```python
from build123d import *

# Parameters (mm, degrees)
F1_DEPTH = 19.05
F2_W     = 6.35
F2_H     = 4.7625
F2_W_2   = 50.8
F3_DEPTH = 63.5
F5_DEPTH = 10.16


with BuildPart() as f1:
    # F0 (on Front) → F1 (new body)
    with BuildSketch(Plane.XZ):
        Polygon((0, -38.1), (0, 0), (0, 38.1), (-38.1, 38.1), (-38.1, 0), (-38.1, -38.1), align=None)
        Polygon((0, 38.1), (0, 0), (0, -38.1), (38.1, -38.1), (38.1, 0), (38.1, 38.1), align=None)
    extrude(amount=F1_DEPTH)

    # F2 (on face) → F3 (cut)
    with BuildSketch(Plane.XY.offset(38.1)):
        Polygon((-25.4, -14.2875), (25.4, -14.2875), (25.4, -9.525), (25.4, -4.7625), (-25.4, -4.7625), (-25.4, -9.525), align=None)
        with Locations((28.575, -11.90625)):
            Rectangle(F2_W, F2_H)
        with Locations((28.575, -7.14375)):
            Rectangle(F2_W, F2_H)
        with Locations((-28.575, -11.90625)):
            Rectangle(F2_W, F2_H)
        with Locations((-28.575, -7.14375)):
            Rectangle(F2_W, F2_H)
        with Locations((0, -16.66875)):
            Rectangle(F2_W_2, F2_H)
    extrude(amount=-F3_DEPTH, mode=Mode.SUBTRACT)

    # F4 (on face) → F5 (cut)
    with BuildSketch(Plane(origin=(0, 0, 0), x_dir=(-1, 0, 0), z_dir=(0, 1, 0))):
        with BuildLine():
            ThreePointArc((-28.956, 19.05), (-25.4, 15.494), (-21.844, 19.05))
            Line((-21.844, 19.05), (-25.4, 19.05))
            Line((-25.4, 19.05), (-28.956, 19.05))
        make_face()
        with BuildLine():
            Line((-25.4, 19.05), (-21.844, 19.05))
            ThreePointArc((-21.844, 19.05), (-25.4, 22.606), (-28.956, 19.05))
            Line((-28.956, 19.05), (-25.4, 19.05))
        make_face()
        with BuildLine():
            ThreePointArc((28.956, 19.05), (25.4, 22.606), (21.844, 19.05))
            Line((21.844, 19.05), (25.4, 19.05))
            Line((25.4, 19.05), (28.956, 19.05))
        make_face()
        with BuildLine():
            Line((25.4, 19.05), (21.844, 19.05))
            ThreePointArc((21.844, 19.05), (25.4, 15.494), (28.956, 19.05))
            Line((28.956, 19.05), (25.4, 19.05))
        make_face()
    extrude(amount=-F5_DEPTH, mode=Mode.SUBTRACT)


solid = f1.part
```
Read the model definition and answer for the solid it produces. Units are mm, in the model's axes. A direction names the side the tool comes from. Coordinates: 2 decimals unless noted, no trailing zeros. Write each loop counter-clockwise with the first axis right and the second up, starting at its lowest first coordinate (ties: lowest second). Pieces come first, ordered by that corner, then holes. Notation, with made-up numbers: (41.5, 40.25) - (99.5, 40.25) arc R27 cw to (99.5, 56.25) - close; hole circle Ø2 at (6, -4). An arc over 180 degrees is marked (long way). Answer as a JSON object with one key per item and string values. Group by question number.
1. A cutting plane is placed at D-D (x = 4). Determine the outline of the cut face in (y, z).
2. Each of these flat-tipped pins is pushed along its axis until it touches: P1, Ø8, axis at x = -21, y = -6, coming from the +Z side; P2, Ø6.5, axis at x = 25.4, z = 19.05, coming from the +Y side; P3, Ø8, axis at x = 10, z = -1.5, coming from the -Y side; P4, Ø10, axis at x = -11, y = -12, coming from the +Z side. Where does it stop, or does it pass through?
3. The mould has two halves that part along Y. Classify faces 6 (the flat face through (-31.75, -9, 7)), 7 (the flat face through (-25.4, -17, 7)), 8 (the flat face through (-1, 0, 1)): +Y half, -Y half, draft (parallel to the pull), parting line (faces both ways), or undercut.
4. A cutting plane is placed at C-C (y = -17). Determine the outline of the cut face in (x, z).
5. A cutting plane is placed at B-B (x = 28). Determine the outline of the cut face in (y, z).
6. Consider L1, parallel to X at y = -14.25, z = 4; L2, parallel to Z at x = 25.4, y = -2.5; L3, parallel to X at y = -14.75, z = -20.5. Determine where each line is inside the solid, lowest interval first. Write a range as [from, to].
7. Which of the six approach directions +Z, -Z, +X, -X, +Y, -Y give full straight-line access (tool end or side, diameter ignored) to faces 1 (the flat face through (-38.1, -9, 1)), 2 (the cylindrical face through (-28.021, -2.348, 16.647)), 3 (the flat face through (25.4, -17, 7)), 4 (the flat face through (38.1, -9, -1)), 5 (the flat face through (29, -14.288, 7))?
8. A cutting plane is placed at A-A (z = 19.05). Determine the outline of the cut face in (x, y).
Worked out:
{
 "1": {"outline": "(-19.05, -38.1) - (0, -38.1) - (0, 38.1) - (-4.76, 38.1) - (-4.76, -25.4) - (-19.05, -25.4) - close"},
 "2": {"P1": "stops at z = 38.1", "P2": "stops at y = -14.29", "P3": "stops at y = -4.76", "P4": "stops at z = -25.4"},
 "3": {"face 6": "undercut", "face 7": "draft", "face 8": "+Y half"},
 "4": {"outline": "(-38.1, -38.1) - (38.1, -38.1) - (38.1, 38.1) - (25.4, 38.1) - (25.4, -25.4) - (-25.4, -25.4) - (-25.4, 38.1) - (-38.1, 38.1) - close"},
 "5": {"outline": "(-19.05, -38.1) - (0, -38.1) - (0, 16.62) - (-4.76, 16.62) - (-4.76, -25.4) - (-14.29, -25.4) - (-14.29, 38.1) - (-19.05, 38.1) - close; (-4.76, 21.48) - (0, 21.48) - (0, 38.1) - (-4.76, 38.1) - close"},
 "6": {"L1": "x = [-38.1, -31.75], [31.75, 38.1]", "L2": "z = [-38.1, 15.49], [22.61, 38.1]", "L3": "x = [-38.1, -25.4], [25.4, 38.1]"},
 "7": {"face 1": "+Z, -Z, -X, +Y, -Y", "face 2": "+Y", "face 3": "+Z, -Y", "face 4": "+Z, -Z, +X, +Y, -Y", "face 5": "+Z"},
 "8": {"outline": "(-38.1, -19.05) - (-25.4, -19.05) - (-25.4, -14.29) - (-31.75, -14.29) - (-31.75, -4.76) - (-28.96, -4.76) - (-28.96, 0) - (-38.1, 0) - close; (-21.84, -4.76) - (21.84, -4.76) - (21.84, 0) - (-21.84, 0) - close; (25.4, -19.05) - (38.1, -19.05) - (38.1, 0) - (28.96, 0) - (28.96, -4.76) - (31.75, -4.76) - (31.75, -14.29) - (25.4, -14.29) - close"}
}
